Verification items for the finished model (mm, model axes). A direction names the side the tool comes from. Give positions to 0.01 mm unless a question says otherwise; leave off trailing zeros. Loops run counter-clockwise (first coordinate to the right, second up) from the corner with the lowest first, then second, coordinate; pieces in that order, holes last. Notation, with made-up numbers: (-13.5, 61.5) -> (15.5, 61.5) arc R37 cw to (15.5, 99.5) -> close; hole circle Ø6 at (-36.75, 72.5). An arc over 180 degrees is marked (long way). Answer in a Markdown table with one row per item. Add a question column.
Q1. Material ranges on probe 1 along X at (y, z) = (1, 8.5); probe 2 along Z at (x, y) = (-18.5, 3.25) (3 decimals); probe 3 along X at (y, z) = (-0.5, 16), recorded low to high.
Q2. Section check A-A on y = -0.5. Give the number of separate pieces and of enclosed holes in the cut face, and give its area (3 significant figures).
Q3. Section check C-C on z = -10.5. Enter the section's corners in (x, y) (3 decimals).
Q4. Set-up check for faces 1 (the face through (-25.4, -3, 0)), 2 (the face through (13, 2, 11.915)): record each of +Z, -Z, +X, -X, +Y, -Y from which the full face is reachable in a straight line by a thin tool's end or side.
Q5. Section check B-B on z = 8. Enter the section's corners in (x, y) (3 decimals).
Q6. Gauge pin test, flat ends, axial feed: P1, Ø1, axis at x = -20, z = 6.5, coming from the +Y side; P2, Ø12, axis at x = 14.5, z = 17, coming from the +Y side. Record the tip position at first contact, or that the pin passes through.
Q7. Release check for a two-part mould opening along X. For faces 3 (the face through (-12, 2, -19.234)), 4 (the face through (23.95, -2.42, 20.7)), 5 (the face through (0, 10.795, -5)) record: pulls with the +X half, pulls with the -X half, needs draft (parallel to the pull), parting line crosses it, or undercut.
```python
from build123d import *

# Parameters (mm, degrees)
F0_W         = 50.8
F0_H         = 44.45
F0_W_2       = 19.05
F0_H_2       = 5.08
F0_W_3       = 21.6944364339
F0_H_3       = 5.4140361476
F1_DEPTH     = 10.795
F2_W         = 50.8
F2_H         = 44.45
F3_DEPTH     = 3.81
F4_R         = 5.08
F5_SIZE      = 1.27
F6_R         = 2.54
F7_R         = 2.53999
F8_T1_DEPTH  = 52.07
F8_T3_DEPTH  = 46.99
F8_T5_DEPTH  = 40.64
F8_T8_ANGLE  = 90
F8_T10_ANGLE = 90


# Not quite as in the source:
# - a fillet or chamfer that OpenCascade refuses, or shapes differently, is made with other operations: its cross-section is extruded or revolved along the edge and cut away or added
# - a fillet or chamfer is up to 0.001 mm smaller than in the source, because OpenCascade refuses the exact size


with BuildPart() as f1:
    # F0 (on Front) → F1 (new body, symmetric)
    with BuildSketch(Plane.XZ):
        Rectangle(F0_W, F0_H)
        with Locations((-11.4416993469, -16.6936574811)):
            Rectangle(F0_W_2, F0_H_2, mode=Mode.SUBTRACT)
        with Locations((-11.4416993469, -9.0736574811)):
            Rectangle(F0_W_2, F0_H_2, mode=Mode.SUBTRACT)
        with Locations((-11.4416993469, -1.4536574811)):
            Rectangle(F0_W_2, F0_H_2, mode=Mode.SUBTRACT)
        with Locations((11.4416993469, -16.6936574811)):
            Rectangle(F0_W_2, F0_H_2, mode=Mode.SUBTRACT)
        with Locations((11.4416993469, -9.0736574811)):
            Rectangle(F0_W_2, F0_H_2, mode=Mode.SUBTRACT)
        with Locations((11.4416993469, -1.4536574811)):
            Rectangle(F0_W_2, F0_H_2, mode=Mode.SUBTRACT)
        with Locations((-11.4416993469, 6.1663425189)):
            Rectangle(F0_W_2, F0_H_2, mode=Mode.SUBTRACT)
        with Locations((-12.7639175639, 14.6224689895)):
            Rectangle(F0_W_3, F0_H_3, mode=Mode.SUBTRACT)
        with Locations((11.4416993469, 6.1663425189)):
            Rectangle(F0_W_2, F0_H_2, mode=Mode.SUBTRACT)
        with Locations((12.7639175639, 14.6224689895)):
            Rectangle(F0_W_3, F0_H_3, mode=Mode.SUBTRACT)
    extrude(amount=F1_DEPTH, both=True)

    # F2 (on face) → F3 (join)
    with BuildSketch(Plane.XZ.offset(10.795)):
        Rectangle(F2_W, F2_H)
    extrude(amount=-F3_DEPTH)

    # F4
    f4_edges = [f1.edges().sort_by_distance(p)[0] for p in [
        (25.4, 0, 22.225),
        (-25.4, 0, 22.225),
    ]]
    fillet(f4_edges, radius=F4_R)

    # F5
    f5_edges = [f1.edges().sort_by_distance(p)[0] for p in [
        (12.763918, 10.795, 11.915451),
        (-12.763918, 10.795, 11.915451),
        (-11.441699, 10.795, 3.626343),
        (11.441699, 10.795, 3.626343),
        (11.441699, 10.795, -3.993657),
        (-11.441699, 10.795, -3.993657),
        (-11.441699, 10.795, -11.613657),
        (11.441699, 10.795, -11.613657),
        (11.441699, 10.795, -19.233657),
        (-11.441699, 10.795, -19.233657),
    ]]
    chamfer(f5_edges, length=F5_SIZE)

    # F6
    f6_edges = [f1.edges().sort_by_distance(p)[0] for p in [
        (11.441699, -6.985, 3.626343),
        (-11.441699, -6.985, 3.626343),
        (-12.763918, -6.985, 11.915451),
        (12.763918, -6.985, 11.915451),
        (11.441699, -6.985, -3.993657),
        (-11.441699, -6.985, -3.993657),
        (11.441699, -6.985, -11.613657),
        (-11.441699, -6.985, -11.613657),
        (11.441699, -6.985, -19.233657),
        (-11.441699, -6.985, -19.233657),
    ]]
    fillet(f6_edges, radius=F6_R)

    # F7 (radius 2.54 in the source; OpenCascade refuses exactly that, so slightly less here)
    f7_edges = [f1.edges().sort_by_distance(p)[0] for p in [
        (11.441699, -6.985, 1.086343),
        (11.441699, -6.985, 8.706343),
        (-11.441699, -6.985, 8.706343),
        (-11.441699, -6.985, 1.086343),
        (-11.441699, -6.985, -6.533657),
        (11.441699, -6.985, -6.533657),
        (-12.763918, -6.985, 17.329487),
        (12.763918, -6.985, 17.329487),
        (11.441699, -6.985, -14.153657),
        (-11.441699, -6.985, -14.153657),
    ]]
    fillet(f7_edges, radius=F7_R)

    # F8: fillet of radius 5.08 on 4 edges, made by hand

    # F8_s2 → F8_t1 (cut)
    with BuildSketch(Plane.XY.offset(-34.925)):
        with BuildLine():
            ThreePointArc((20.32, 10.795), (23.9121024484, 9.3071024484), (25.4, 5.715))
            Line((25.4, 5.715), (25.4, 10.795))
            Line((25.4, 10.795), (20.32, 10.795))
        make_face()
        with BuildLine():
            ThreePointArc((-20.32, 10.795), (-23.9121024484, 9.3071024484), (-25.4, 5.715))
            Line((-25.4, 5.715), (-25.4, 10.795))
            Line((-25.4, 10.795), (-20.32, 10.795))
        make_face()
    extrude(amount=F8_T1_DEPTH, mode=Mode.SUBTRACT)

    # F8_s4 → F8_t3 (cut)
    with BuildSketch(Plane.XZ.offset(-23.495)):
        with BuildLine():
            ThreePointArc((-25.4, -17.145), (-23.9121024484, -20.7371024484), (-20.32, -22.225))
            Line((-20.32, -22.225), (-25.4, -22.225))
            Line((-25.4, -22.225), (-25.4, -17.145))
        make_face()
        with BuildLine():
            ThreePointArc((20.32, -22.225), (23.9121024484, -20.7371024484), (25.4, -17.145))
            Line((25.4, -17.145), (25.4, -22.225))
            Line((25.4, -22.225), (20.32, -22.225))
        make_face()
    extrude(amount=F8_T3_DEPTH, mode=Mode.SUBTRACT)

    # F8_s6 → F8_t5 (cut)
    with BuildSketch(Plane.YZ.offset(-20.32)):
        with BuildLine():
            ThreePointArc((10.795, 17.145), (9.3071024484, 20.7371024484), (5.715, 22.225))
            Line((5.715, 22.225), (10.795, 22.225))
            Line((10.795, 22.225), (10.795, 17.145))
        make_face()
    extrude(amount=F8_T5_DEPTH, mode=Mode.SUBTRACT)

    # F8_s7 → F8_t8 (revolve, cut)
    with BuildSketch(Plane.XY.offset(17.145)):
        with BuildLine():
            ThreePointArc((-20.32, 10.795), (-23.9121024484, 9.3071024484), (-25.4, 5.715))
            Line((-25.4, 5.715), (-25.4, 10.795))
            Line((-25.4, 10.795), (-20.32, 10.795))
        make_face()
    revolve(axis=Axis((-20.32, 10.795, 17.145), (0, 1, 0)), revolution_arc=F8_T8_ANGLE, mode=Mode.SUBTRACT)

    # F8_s9 → F8_t10 (revolve, cut)
    with BuildSketch(Plane.YZ.offset(20.32)):
        with BuildLine():
            ThreePointArc((10.795, 17.145), (9.3071024484, 20.7371024484), (5.715, 22.225))
            Line((5.715, 22.225), (10.795, 22.225))
            Line((10.795, 22.225), (10.795, 17.145))
        make_face()
    revolve(axis=Axis((20.32, 10.795, 17.145), (0, 1, 0)), revolution_arc=F8_T10_ANGLE, mode=Mode.SUBTRACT)


solid = f1.part
```
Taken from the geometry:
| question | item | result |
|---|---|---|
| 1 | probe 1 | x = -25.4 to -20.97, -1.92 to 1.92, 20.97 to 25.4 |
| 1 | probe 2 | z = -22.225 to -19.234, -14.154 to -11.614, -6.534 to -3.994, 1.086 to 3.626, 8.706 to 11.915, 17.329 to 22.225 |
| 1 | probe 3 | x = -25.4 to -23.61, -1.92 to 1.92, 23.61 to 25.4 |
| 2 | separate pieces | 1 |
| 2 | enclosed holes | 10 |
| 2 | area | 1,230 mm² |
| 3 | outline | (-25.4, -10.795) -> (25.4, -10.795) -> (25.4, 5.715) arc R5.08 ccw to (20.967, 10.754) -> (20.967, -6.547) -> (1.917, -6.547) -> (1.917, 10.795) -> (-1.917, 10.795) -> (-1.917, -6.547) -> (-20.967, -6.547) -> (-20.967, 10.754) arc R5.08 ccw to (-25.4, 5.715) -> close |
| 4 | face 1 | +Z, -Z, -X, +Y, -Y |
| 4 | face 2 | +Y |
| 5 | outline | (-25.4, -10.795) -> (25.4, -10.795) -> (25.4, 5.715) arc R5.08 ccw to (20.967, 10.754) -> (20.967, -6.203) -> (1.917, -6.203) -> (1.917, 10.795) -> (-1.917, 10.795) -> (-1.917, -6.203) -> (-20.967, -6.203) -> (-20.967, 10.754) arc R5.08 ccw to (-25.4, 5.715) -> close |
| 6 | P1 | stops at y = -6.84 |
| 6 | P2 | stops at y = 10.79 |
| 7 | face 3 | undercut |
| 7 | face 4 | pulls with the +X half |
| 7 | face 5 | needs draft |
